```python
from build123d import *

# Parameters (mm, degrees)
ESBO_O1_W                = 166
ESBO_O1_H                = 120
RESSALTO_EXTRUS_O1_DEPTH = 6
ESBO_O2_R                = 3.5
CORTE_EXTRUS_O1_DEPTH    = 103.591422643
ESBO_O3_W                = 80
ESBO_O3_H                = 80
RESSALTO_EXTRUS_O2_DEPTH = 6
FILETE1_R                = 10
CHANFRO1_SIZE            = 6
CORTE_EXTRUS_O2_DEPTH    = 10
CORTE_EXTRUS_O3_DEPTH    = 131.096118313
RESSALTO_EXTRUS_O3_DEPTH = 6
FILETE2_R                = 10
CHANFRO2_SIZE            = 5
FILETE3_R                = 1


with BuildPart() as part:
    # Esboço1 → Ressalto-extrusão1 (new body)
    with BuildSketch(Plane.XY):
        Rectangle(ESBO_O1_W, ESBO_O1_H)
    extrude(amount=RESSALTO_EXTRUS_O1_DEPTH)

    # Esboço2 → Corte-extrusão1 (cut, through all)
    with BuildSketch(Plane.XY.offset(6)):
        with Locations((-63.75, -51.4)):
            Circle(ESBO_O2_R)
        with Locations((-63.75, -26)):
            Circle(ESBO_O2_R)
        with Locations((-63.75, 26)):
            Circle(ESBO_O2_R)
        with Locations((-63.75, 51.4)):
            Circle(ESBO_O2_R)
        with Locations((63.75, -51.4)):
            Circle(ESBO_O2_R)
        with Locations((63.75, -26)):
            Circle(ESBO_O2_R)
        with Locations((63.75, 26)):
            Circle(ESBO_O2_R)
        with Locations((63.75, 51.4)):
            Circle(ESBO_O2_R)
    extrude(amount=-CORTE_EXTRUS_O1_DEPTH, mode=Mode.SUBTRACT)

    # Esboço3 → Ressalto-extrusão2 (add, through all)
    with BuildSketch(Plane.XY.offset(6)):
        with Locations((0, -60)):
            Rectangle(ESBO_O3_W, ESBO_O3_H)
    extrude(amount=-RESSALTO_EXTRUS_O2_DEPTH)

    # Filete1
    filete1_edges = [part.edges().sort_by_distance(p)[0] for p in [
        (40, -60, 3),
        (-40, -60, 3),
    ]]
    fillet(filete1_edges, radius=FILETE1_R)

    # Chanfro1
    chanfro1_edges = [part.edges().sort_by_distance(p)[0] for p in [
        (-40, -100, 3),
        (40, -100, 3),
    ]]
    chamfer(chanfro1_edges, length=CHANFRO1_SIZE)

    # Esboço4 → Corte-extrusão2 (cut)
    with BuildSketch(Plane.XY.offset(6)):
        with BuildLine():
            Line((-19.5, -2), (-19.5, -88))
            ThreePointArc((-19.5, -88), (-23, -91.5), (-26.5, -88))
            Line((-26.5, -88), (-26.5, -2))
            ThreePointArc((-26.5, -2), (-23, 1.5), (-19.5, -2))
        make_face()
        with BuildLine():
            Line((26.5, -2), (26.5, -88))
            ThreePointArc((26.5, -88), (23, -91.5), (19.5, -88))
            Line((19.5, -88), (19.5, -2))
            ThreePointArc((19.5, -2), (23, 1.5), (26.5, -2))
        make_face()
    extrude(amount=-CORTE_EXTRUS_O2_DEPTH, mode=Mode.SUBTRACT)

    # Esboço5 → Corte-extrusão3 (cut, through all)
    with BuildSketch(Plane.XY.offset(6)):
        Polygon((-51.75, 52), (-51.75, 14), (-75, 14), (-75, -14), (-51.75, -14), (-51.75, -42), (-35.75, -42), (-35.75, 14), (-11.75, 14), (-11.75, 52), align=None)
        Polygon((75, -14), (51.75, -14), (51.75, -42), (35.75, -42), (35.75, 14), (11.75, 14), (11.75, 52), (51.75, 52), (51.75, 14), (75, 14), align=None)
    extrude(amount=-CORTE_EXTRUS_O3_DEPTH, mode=Mode.SUBTRACT)

    # Esboço6 → Ressalto-extrusão3 (add, through all)
    with BuildSketch(Plane.XY.offset(6)):
        Polygon((-51.75, 14), (-35.75, -2), (-35.75, 14), (-51.75, 30), align=None)
        Polygon((35.75, 14), (51.75, 30), (51.75, 14), (35.75, -2), align=None)
    extrude(amount=-RESSALTO_EXTRUS_O3_DEPTH)

    # Filete2
    filete2_edges = [part.edges().sort_by_distance(p)[0] for p in [
        (-51.75, -14, 3),
        (51.75, -14, 3),
    ]]
    fillet(filete2_edges, radius=FILETE2_R)

    # Chanfro2
    chanfro2_edges = [part.edges().sort_by_distance(p)[0] for p in [
        (-51.75, 52, 3),
        (-11.75, 52, 3),
        (-11.75, 14, 3),
        (-35.75, -42, 3),
        (-51.75, -42, 3),
        (-75, -14, 3),
        (-75, 14, 3),
        (75, 14, 3),
        (75, -14, 3),
        (51.75, -42, 3),
        (35.75, -42, 3),
        (11.75, 14, 3),
        (11.75, 52, 3),
        (51.75, 52, 3),
    ]]
    chamfer(chanfro2_edges, length=CHANFRO2_SIZE)

    # Filete3
    filete3_edges = [part.edges().sort_by_distance(p)[0] for p in [
        (83, -60, 3),
        (-83, -60, 3),
        (-83, 60, 3),
        (83, 60, 3),
    ]]
    fillet(filete3_edges, radius=FILETE3_R)


solid = part.part
```
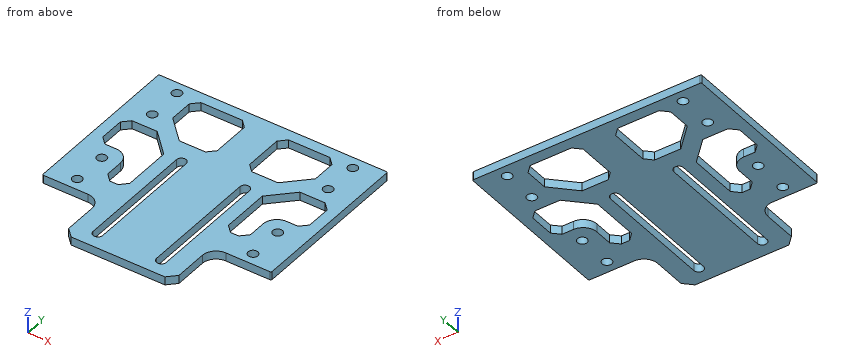
Could you check a few things on this model? Use its own coordinates, in mm. Give positions to 0.01 mm unless a question says otherwise; leave off trailing zeros. Order: outer loops, then holes, each group sorted by start corner. A loop starts at its lowest first (then second) coordinate and runs counter-clockwise, first axis right, second up.
Q1. Suppose I cut it at D-D, the plane y = -26. Write out the boundary of the cut face in (x, z), and give its area (3 significant figures).
Q2. Suppose I cut it at C-C, the plane y = 17. Write out the boundary of the cut face in (x, z), and give its area (3 significant figures).
Q3. Suppose I cut it at B-B, the plane x = -63.75. Write out the boundary of the cut face in (y, z), and give its area (3 significant figures).
Q4. Suppose I cut it at A-A, the plane y = -51.4. Write out the boundary of the cut face in (x, z).
Q5. If I drill on line 1 along Y through (x, z) = (63.75, 3.25); line 2 along X through (y, z) = (3, 2.75); line 3 along X through (y, z) = (39, 1), over which ranges is the centre line in solid material (lowest first)?
Q6. I'm going to push flat-ended pins straight in: P1, Ø12, axis at x = 21, y = -2.5, coming from the +Z side; P2, Ø6.5, axis at x = 63.75, y = 26, coming from the +Z side. Where does each tip first touch, or does it pass through?
Solution:
1. outline: (-83, 0) - (-67.25, 0) - (-67.25, 6) - (-83, 6) - close; (-60.25, 0) - (-51.75, 0) - (-51.75, 6) - (-60.25, 6) - close; (-35.75, 0) - (-26.5, 0) - (-26.5, 6) - (-35.75, 6) - close; (-19.5, 0) - (19.5, 0) - (19.5, 6) - (-19.5, 6) - close; (26.5, 0) - (35.75, 0) - (35.75, 6) - (26.5, 6) - close; (51.75, 0) - (60.25, 0) - (60.25, 6) - (51.75, 6) - close; (67.25, 0) - (83, 0) - (83, 6) - (67.25, 6) - close
1. area: 636 mm2
2. outline: (-83, 0) - (-38.75, 0) - (-38.75, 6) - (-83, 6) - close; (-13.75, 0) - (13.75, 0) - (13.75, 6) - (-13.75, 6) - close; (38.75, 0) - (83, 0) - (83, 6) - (38.75, 6) - close
2. area: 696 mm2
3. outline: (-60, 0) - (-54.9, 0) - (-54.9, 6) - (-60, 6) - close; (-47.9, 0) - (-29.5, 0) - (-29.5, 6) - (-47.9, 6) - close; (-22.5, 0) - (-14, 0) - (-14, 6) - (-22.5, 6) - close; (14, 0) - (22.5, 0) - (22.5, 6) - (14, 6) - close; (29.5, 0) - (47.9, 0) - (47.9, 6) - (29.5, 6) - close; (54.9, 0) - (60, 0) - (60, 6) - (54.9, 6) - close
3. area: 384 mm2
4. outline: (-83, 0) - (-67.25, 0) - (-67.25, 6) - (-83, 6) - close; (-60.25, 0) - (-26.5, 0) - (-26.5, 6) - (-60.25, 6) - close; (-19.5, 0) - (19.5, 0) - (19.5, 6) - (-19.5, 6) - close; (26.5, 0) - (60.25, 0) - (60.25, 6) - (26.5, 6) - close; (67.25, 0) - (83, 0) - (83, 6) - (67.25, 6) - close
5. line 1: y = -60 to -54.9, -47.9 to -29.5, -22.5 to -14, 14 to 22.5, 29.5 to 47.9, 54.9 to 60
5. line 2: x = -83 to -75, -40.75 to 40.75, 75 to 83
5. line 3: x = -83 to -51.75, -11.75 to 11.75, 51.75 to 83
6. P1: stops at z = 6
6. P2: passes through
